CAD build for the part. Positions are in the model's coordinates, mm. A direction names the side the tool comes from. Give positions to 0.01 mm unless a question says otherwise; leave off trailing zeros. Order: outer loops, then holes, each group sorted by start corner. A loop starts at its lowest first (then second) coordinate and runs counter-clockwise, first axis right, second up. Notation, with made-up numbers: M 58,14 L 74,14 A29 ccw 74,40 Z; hole C -22,-7 d1. An arc over 180 degrees is marked long. Put each result on its own line as item: value. Start each with the question number.
1) Cut at C-C (z = 11). Write the cut outline in (x, y), and give its area (3 significant figures).
2) Two-plate mould, pull along X, no slides. Class faces 3 (the face through (0, 0, 6)), 4 (the face through (-22, 4, 6)), 5 (the face through (22, 4, 6)), 6 (the face through (-21.5, 4, 6)): released by +X, released by -X, zero draft, split by the parting line, or undercut.
3) Cut at D-D (x = -3). Write the cut outline in (y, z).
4) Drill centre lines: line 1 (X direction, y = 2.5, z = 10.5); line 2 (Y direction, x = -5, z = 2.75). Where is each one in solid material? Low to high. Write a range as [from, to].
5) Cut at B-B (y = 7). Write the cut outline in (x, z), and give its area (3 significant figures).
6) Tool access for faces 1 (the face through (21.5, 4, 6)), 2 (the face through (0.1, -0.3, 0)): list every direction of +Z, -Z, +X, -X, +Y, -Y with a clear straight run to the whole face (end or side of a thin tool).
7) Pin check, flat tips, straight feed: pin 1 (2 mm diameter, centred on x = 7, y = 2, fed in from +Z); pin 2 (5 mm diameter, centred on x = -13, z = 7, fed in from +Y). Stop position of each tip, or through.
8) Cut at A-A (z = 7). Write the cut outline in (x, y), and give its area (3 significant figures).
```python
from build123d import *

# Parameters (mm, degrees)
BOSS_EXTRUDE1_DEPTH = 12
SKETCH2_W           = 6
SKETCH2_H           = 1.5
CUT_EXTRUDE1_DEPTH  = 45


with BuildPart() as part:
    # Sketch1 → Boss-Extrude1 (new body)
    with BuildSketch(Plane.XY):
        with BuildLine():
            Line((-21.5, 7.5), (-21.5, 0.49))
            ThreePointArc((-21.5, 0.49), (-21.356482323, 0.143517677), (-21.01, 0))
            Line((-21.01, 0), (0, 0))
            Line((0, 0), (21.01, 0))
            ThreePointArc((21.01, 0), (21.356482323, 0.143517677), (21.5, 0.49))
            Line((21.5, 0.49), (21.5, 7.5))
            Line((21.5, 7.5), (22, 7.5))
            Line((22, 7.5), (22, -0.01))
            ThreePointArc((22, -0.01), (21.856482323, -0.356482323), (21.51, -0.5))
            Line((21.51, -0.5), (-21.51, -0.5))
            ThreePointArc((-21.51, -0.5), (-21.856482323, -0.356482323), (-22, -0.01))
            Line((-22, -0.01), (-22, 7.5))
            Line((-22, 7.5), (-21.5, 7.5))
        make_face()
    extrude(amount=BOSS_EXTRUDE1_DEPTH)

    # Sketch2 → Cut-Extrude1 (cut, through all)
    with BuildSketch(Plane.ZY.offset(22)):
        with Locations((6, 5.3)):
            Rectangle(SKETCH2_W, SKETCH2_H)
    extrude(amount=-CUT_EXTRUDE1_DEPTH, mode=Mode.SUBTRACT)


solid = part.part
```
Solution:
1. outline: M -22,-0.01 A0.49 ccw -21.51,-0.5 L 21.51,-0.5 A0.49 ccw 22,-0.01 L 22,7.5 L 21.5,7.5 L 21.5,0.49 A0.49 cw 21.01,0 L -21.01,0 A0.49 cw -21.5,0.49 L -21.5,7.5 L -22,7.5 Z
1. area: 29.5 mm²
2. face 3: undercut
2. face 4: released by -X
2. face 5: released by +X
2. face 6: undercut
3. outline: M -0.5,0 L 0,0 L 0,12 L -0.5,12 Z
4. line 1: [-22, -21.5], [21.5, 22]
4. line 2: [-0.5, 0]
5. outline: M -22,0 L -21.5,0 L -21.5,12 L -22,12 Z; M 21.5,0 L 22,0 L 22,12 L 21.5,12 Z
5. area: 12.0 mm²
6. face 1: +Z, -Z, +Y
6. face 2: -Z, +X, -X, +Y, -Y
7. pin 1: through
7. pin 2: y = 0
8. outline: M -22,-0.01 A0.49 ccw -21.51,-0.5 L 21.51,-0.5 A0.49 ccw 22,-0.01 L 22,4.55 L 21.5,4.55 L 21.5,0.49 A0.49 cw 21.01,0 L -21.01,0 A0.49 cw -21.5,0.49 L -21.5,4.55 L -22,4.55 Z; M -22,6.05 L -21.5,6.05 L -21.5,7.5 L -22,7.5 Z; M 21.5,6.05 L 22,6.05 L 22,7.5 L 21.5,7.5 Z
8. area: 28.0 mm²
